Geometry: final body of the model. Coordinates: model frame, mm. Face numbers are marked on the shaded views. A direction names the side the tool comes from. Give positions to 0.01 mm unless a question says otherwise; leave off trailing zeros. Write each loop counter-clockwise with the first axis right and the second up, starting at its lowest first coordinate (ties: lowest second). Pieces come first, ordered by that corner, then holes. Notation, with made-up numbers: (0.25, -36.75) -> (5.25, -36.75) arc R32 ccw to (5.25, -9.75) -> close; hole circle Ø10 at (-7, -5). An arc over 180 degrees is marked (long way). Answer as a JSON object with one key per item and string values. Group by question number.
(1) Section query C-C on x = -16.5. Output: boundary loops of the cut face in (y, z).
(2) Section query D-D on z = -18.5. Output: boundary loops of the cut face in (x, y).
(3) Material intervals for probe 1 along Z at (x, y) = (-24, -3); probe 2 along X at (y, z) = (-3.25, -24.5); probe 3 along Z at (x, y) = (-3, -3), sorted ascending.
(4) Contact query for flat-ended pins moving along their axis: pin 1 Ø3 at (y, z) = (-5, -22) entering from -X; pin 2 Ø3 at (y, z) = (-1.5, -2.5) entering from +X; pin 3 Ø1.5 at (x, y) = (4.5, -3.5) entering from -Z. Output: stop coordinate, or through.
(5) Set-up query: the marked faces 4 and 5. Return all of +Z, -Z, +X, -X, +Y, -Y with unobstructed straight access to the full face (end or side cutting, diameter ignored); none if empty.
(6) Section query B-B on z = 30.5. Output: boundary loops of the cut face in (x, y).
(7) Draft query along X for the marked faces 1, 2 and 3. Return one class per face: +X half, -X half, draft (parallel to the pull), parting line (faces both ways), or undercut.
(8) Section query A-A on y = -1.25. Output: boundary loops of the cut face in (x, z) (3 decimals), plus the area to 3 significant figures.
from build123d import *

# Parameters (mm, degrees)
F0_R     = 37.049444
F1_DEPTH = 6.35


with BuildPart() as f1:
    # F0 (on Front) → F1 (new body)
    with BuildSketch(Plane.XZ):
        Circle(F0_R)
        with BuildLine():
            ThreePointArc((32.775383, 8.520914), (33.591419, 4.295144), (33.864904, 0))
            ThreePointArc((33.864904, 0), (27.812587, -19.320759), (11.818969, -31.735527))
            ThreePointArc((11.818969, -31.735527), (9.491898, -32.507469), (7.115076, -33.109023))
            ThreePointArc((7.115076, -33.109023), (-0.041069, -33.864879), (-7.19536, -33.091668))
            ThreePointArc((-7.19536, -33.091668), (-9.531315, -32.495934), (-11.818969, -31.735527))
            ThreePointArc((-11.818969, -31.735527), (-30.038464, -15.637212), (-32.775383, 8.520914))
            ThreePointArc((-32.775383, 8.520914), (-30.241055, 15.241729), (-26.346281, 21.276869))
            ThreePointArc((-26.346281, 21.276869), (-23.481444, 24.401916), (-20.248603, 27.144535))
            ThreePointArc((-20.248603, 27.144535), (-16.503137, 29.571577), (-12.471031, 31.484998))
            ThreePointArc((-12.471031, 31.484998), (0, 33.864904), (12.471031, 31.484998))
            ThreePointArc((12.471031, 31.484998), (16.970465, 29.305887), (21.100053, 26.4881))
            ThreePointArc((21.100053, 26.4881), (24.733428, 23.131996), (27.839175, 19.282428))
            ThreePointArc((27.839175, 19.282428), (30.781223, 14.119065), (32.775383, 8.520914))
        make_face(mode=Mode.SUBTRACT)
        with BuildLine():
            Line((11.818969, -31.735527), (32.775383, 8.520914))
            ThreePointArc((32.775383, 8.520914), (30.781223, 14.119065), (27.839175, 19.282428))
            Line((27.839175, 19.282428), (11.500335, -10.058812))
            Line((11.500335, -10.058812), (6.35, 0))
            Line((6.35, 0), (-6.35, 0))
            Line((-6.35, 0), (-9.970913, -10.704888))
            Line((-9.970913, -10.704888), (-26.346281, 21.276869))
            ThreePointArc((-26.346281, 21.276869), (-30.241055, 15.241729), (-32.775383, 8.520914))
            Line((-32.775383, 8.520914), (-11.818969, -31.735527))
            ThreePointArc((-11.818969, -31.735527), (-9.531315, -32.495934), (-7.19536, -33.091668))
            Line((-7.19536, -33.091668), (0, -22.65686))
            Line((0, -22.65686), (7.115076, -33.109023))
            ThreePointArc((7.115076, -33.109023), (9.491898, -32.507469), (11.818969, -31.735527))
        make_face()
        with BuildLine():
            Line((6.35, 0), (21.100053, 26.4881))
            ThreePointArc((21.100053, 26.4881), (16.970465, 29.305887), (12.471031, 31.484998))
            Line((12.471031, 31.484998), (0, 8.249764))
            Line((0, 8.249764), (-12.471031, 31.484998))
            ThreePointArc((-12.471031, 31.484998), (-16.503137, 29.571577), (-20.248603, 27.144535))
            Line((-20.248603, 27.144535), (-6.35, 0))
            Line((-6.35, 0), (6.35, 0))
        make_face()
    extrude(amount=F1_DEPTH)


solid = f1.part
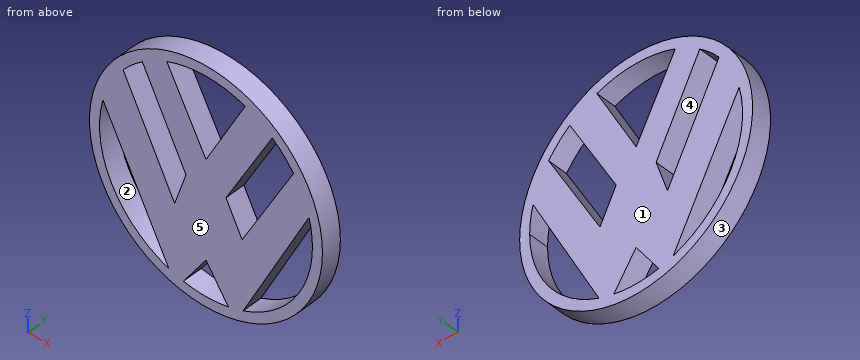
Answer list:
{
 "1": {"outline": "(-6.35, -33.17) -> (0, -33.17) -> (0, -29.57) -> (-6.35, -29.57) -> close; (-6.35, -22.74) -> (0, -22.74) -> (0, 2.05) -> (-6.35, 2.05) -> close; (-6.35, 19.82) -> (0, 19.82) -> (0, 33.17) -> (-6.35, 33.17) -> close"},
 "2": {"outline": "(-32.1, -6.35) -> (-28.37, -6.35) -> (-28.37, 0) -> (-32.1, 0) -> close; (-18.71, -6.35) -> (18.71, -6.35) -> (18.71, 0) -> (-18.71, 0) -> close; (28.37, -6.35) -> (32.1, -6.35) -> (32.1, 0) -> (28.37, 0) -> close"},
 "3": {"probe 1": "-28.23 to -23.89, -8.34 to 16.69, 23.89 to 28.23", "probe 2": "-27.79 to -23.38, -15.59 to -1.27, 1.25 to 15.59, 23.38 to 27.79", "probe 3": "-36.93 to -33.73, -27.01 to 13.84, 33.73 to 36.93"},
 "4": {"pin 1": "x = -30.86", "pin 2": "x = 37.04", "pin 3": "z = -36.86"},
 "5": {"face 4": "+Y, -Y", "face 5": "+Z, -Z, +X, -X, -Y"},
 "6": {"outline": "(-21.03, -6.35) -> (-11.94, -6.35) -> (-11.94, 0) -> (-21.03, 0) -> close; (11.94, -6.35) -> (21.03, -6.35) -> (21.03, 0) -> (11.94, 0) -> close"},
 "7": {"face 1": "draft", "face 2": "undercut", "face 3": "parting line"},
 "8": {"outline": "circle Ø74.099 at (0, 0); hole (-32.775, 8.521) arc R33.865 ccw to (-11.819, -31.736) -> close; hole (-26.346, 21.277) -> (-9.971, -10.705) -> (-6.35, 0) -> (-20.249, 27.145) arc R33.865 ccw to start; hole (-12.471, 31.485) -> (0, 8.25) -> (12.471, 31.485) arc R33.865 ccw to start; hole (-7.195, -33.092) arc R33.865 ccw to (7.115, -33.109) -> (0, -22.657) -> close; hole (6.35, 0) -> (11.5, -10.059) -> (27.839, 19.282) arc R33.865 ccw to (21.1, 26.488) -> close; hole (11.819, -31.736) arc R33.865 ccw to (33.865, 0) arc R33.865 ccw to (32.775, 8.521) -> close", "area": "2,780 mm2"}
}
